Autodesk Inventor part; units mm, degrees
ref_plane "YZ Plane" through (0, 0, 0) normal (1, 0, 0) x (0, 1, 0)
ref_plane "XZ Plane" through (0, 0, 0) normal (0, 1, 0) x (-1, 0, 0)
ref_plane "XY Plane" through (0, 0, 0) normal (0, 0, 1) x (1, 0, 0)
sketch "Sketch1" plane through (0, 0, 0) normal (0, 1, 0) x (-1, 0, 0)
  line L0 (0, 10.6093) -> (-18, 10.6093)
  line L1 (-18, 10.6093) -> (-18, -18.3907)
  line L2 (-18, -18.3907) -> (0, -18.3907)
  line L3 (0, -15.8907) -> (6, -15.8907)
  line L4 (6, -15.8907) -> (6, -6.8907)
  line L5 (6, -6.8907) -> (0, -6.8907)
  line L6 (0, -6.8907) -> (0, -15.8907)
  line L7 (0, -3.8907) -> (-9, -3.8907) construction
  line L8 (-9, -18.3907) -> (-9, 10.6093) construction
  line L9 (0, 8.1093) -> (6, 8.1093)
  line L10 (6, 8.1093) -> (6, -0.8907)
  line L11 (6, -0.8907) -> (0, -0.8907)
  line L12 (0, -0.8907) -> (0, 8.1093)
  line L13 (-18, -15.8907) -> (-24, -15.8907)
  line L14 (-24, -15.8907) -> (-24, -6.8907)
  line L15 (-24, -6.8907) -> (-18, -6.8907)
  line L16 (-18, -6.8907) -> (-18, -15.8907)
  line L17 (-18, 8.1093) -> (-24, 8.1093)
  line L18 (-24, 8.1093) -> (-24, -0.8907)
  line L19 (-24, -0.8907) -> (-18, -0.8907)
  line L20 (-18, -0.8907) -> (-18, 8.1093)
  line L21 (0, -15.8907) -> (0, 8.1093)
  line L22 (-9, -3.8907) -> (-18, -3.8907) construction
  line L23 (0, -18.3907) -> (0, 10.6093)
  dimension "d49" = 18
  dimension "d50" = 29
  dimension "d54" = 9
  dimension "d60" = 6
  dimension "d76" = 6
  dimension "d87" = 30
extrude "Extrusion1" add sketch "Sketch1" along normal blind 6
sketch "Sketch3" plane through (0, 6, 0) normal (0, 1, 0) x (1, 0, 0)
  line L0 (18, 18.3907) -> (0, 18.3907) construction
  line L1 (9, 18.3907) -> (9, -10.6093) construction
  line L2 (0, -10.6093) -> (18, -10.6093) construction
  line L3 (0, 0.8907) -> (0, 6.8907) construction
  line L4 (0, 3.8907) -> (18, 3.8907) construction
  line L5 (18, 0.8907) -> (18, 6.8907) construction
  circle A0 centre (9, 12.3907) radius 1
  circle A1 centre (9, -4.6093) radius 1
  circle A2 centre (9, 3.8907) radius 3
  point P0 (0, 0)
  dimension "d91" = 2
  dimension "d92" = 8.5
  dimension "d96" = 6
extrude "Extrusion3" cut sketch "Sketch3" against normal through all
properties part number "thumper-bumper-top-v3"
Design review of the part built by this model. Coordinates are the model's own, in mm. A direction names the side the tool comes from. Coordinates: 2 decimals unless noted, no trailing zeros. Loops run counter-clockwise (first coordinate to the right, second up) from the corner with the lowest first, then second, coordinate; pieces in that order, holes last. Notation, with made-up numbers: (68, 31.5) - (72, 31.5) arc R9 ccw to (72, 45.5) - close; hole circle Ø4 at (82, 84). An arc over 180 degrees is marked (long way). Use CSV: the item, a comma, the result in double quotes. Start each with the question number.
1. Add section A-A on x = 9. Give the boundary of the cut face in (y, z).
2. To check wall thickness, follow probe 1 along Z at (x, y) = (9, 2.3); probe 2 along X at (y, z) = (5.7, -3.75); probe 3 along X at (y, z) = (1.7, 8.75). State the ranges of each line that lie inside material, in increasing order.
3. Add section B-B on z = -2.5. Give the boundary of the cut face in (x, y).
4. Clearance check with flat-ended pins moving along their axes: pin 1 (1.8 mm diameter, centred on x = -2.5, y = 2.5, fed in from +Z); pin 2 (3 mm diameter, centred on x = 21, y = 4, fed in from -Z); pin 3 (2 mm diameter, centred on y = 3, z = 9.5, fed in from +X). State where each tip first meets the part, or that it passes through.
5. For faces 1 (the flat face through (-3, 3, -6.891)), 2 (the flat face through (0, 3, 9)), 3 (the flat face through (0, 3, -17)), list the 3-axis set-ups (+Z, -Z, +X, -X, +Y, -Y) from which the entire face can be reached by the end or side of a thin tool; tool diameter is ignored.
6. Mouldability with a two-part tool opening along Z and no side actions: class faces 4 (the flat face through (9, 3, 10.609)), 5 (the flat face through (-6, 3, -11)), 6 (the flat face through (18, 3, -4)) as released by +Z, released by -Z, zero draft, split by the parting line, or undercut.
7. Add section D-D on y = 2.35. Give the boundary of the cut face in (x, z).
8. Add section C-C on x = 21.5. Give the boundary of the cut face in (y, z).
Resolved:
1,outline,"(0, -18.39) - (6, -18.39) - (6, -13.39) - (0, -13.39) - close; (0, -11.39) - (6, -11.39) - (6, -6.89) - (0, -6.89) - close; (0, -0.89) - (6, -0.89) - (6, 3.61) - (0, 3.61) - close; (0, 5.61) - (6, 5.61) - (6, 10.61) - (0, 10.61) - close"
2,probe 1,"-18.39 to -13.39, -11.39 to -6.89, -0.89 to 3.61, 5.61 to 10.61"
2,probe 2,"0 to 6, 12 to 18"
2,probe 3,"0 to 18"
3,outline,"(0, 0) - (6.34, 0) - (6.34, 6) - (0, 6) - close; (11.66, 0) - (18, 0) - (18, 6) - (11.66, 6) - close"
4,pin 1,"z = 8.11"
4,pin 2,"z = -15.89"
4,pin 3,"x = 18"
5,face 1,"-X, +Y, -Y"
5,face 2,"+Z, -X, +Y, -Y"
5,face 3,"-Z, -X, +Y, -Y"
6,face 4,"released by +Z"
6,face 5,"zero draft"
6,face 6,"undercut"
7,outline,"(-6, -15.89) - (0, -15.89) - (0, -18.39) - (18, -18.39) - (18, -15.89) - (24, -15.89) - (24, -6.89) - (18, -6.89) - (18, -0.89) - (24, -0.89) - (24, 8.11) - (18, 8.11) - (18, 10.61) - (0, 10.61) - (0, 8.11) - (-6, 8.11) - (-6, -0.89) - (0, -0.89) - (0, -6.89) - (-6, -6.89) - close; hole circle Ø6 at (9, -3.89); hole circle Ø2 at (9, -12.39); hole circle Ø2 at (9, 4.61)"
8,outline,"(0, -15.89) - (6, -15.89) - (6, -6.89) - (0, -6.89) - close; (0, -0.89) - (6, -0.89) - (6, 8.11) - (0, 8.11) - close"
